Design review of the part built by this model. Coordinates are the model's own, in mm. Face numbers are marked on the shaded views. A direction names the side the tool comes from. Coordinates: 2 decimals unless noted, no trailing zeros. Order: outer loops, then holes, each group sorted by start corner. A loop starts at its lowest first (then second) coordinate and runs counter-clockwise, first axis right, second up. Notation, with made-up numbers: M 31,6.25 L 68,6.25 A14 ccw 68,22.25 Z; hole C -34,5.5 d7. An arc over 180 degrees is marked long. Use CSV: the item, a comma, the result in double quotes.
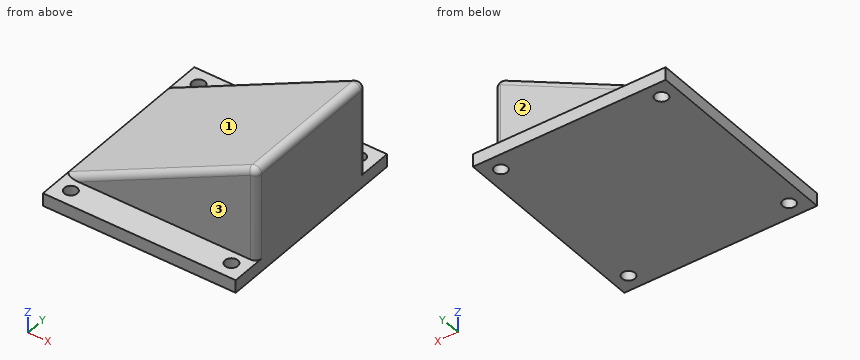
```python
from build123d import *

# Parameters (mm, degrees)
F0_W     = 30
F0_H     = 32
F1_DEPTH = 2
F2_R     = 1
F3_DEPTH = 2
F4_W     = 30
F4_H     = 23
F5_DEPTH = 15
F7_DEPTH = 23
F8_R     = 1


with BuildPart() as f1:
    # F0 (on Top) → F1 (new body)
    with BuildSketch(Plane.XY):
        Rectangle(F0_W, F0_H)
    extrude(amount=F1_DEPTH)

    # F2 (on face) → F3 (cut)
    with BuildSketch(Plane.XY.offset(2)):
        with Locations((12.5, 13.5)):
            Circle(F2_R)
        with Locations((-12.5, 13.5)):
            Circle(F2_R)
        with Locations((-12.5, -13.5)):
            Circle(F2_R)
        with Locations((12.5, -13.5)):
            Circle(F2_R)
    extrude(amount=-F3_DEPTH, mode=Mode.SUBTRACT)

    # F4 (on face) → F5 (join)
    with BuildSketch(Plane.XY.offset(2)):
        Rectangle(F4_W, F4_H)
    extrude(amount=F5_DEPTH)

    # F6 (on face) → F7 (cut)
    with BuildSketch(Plane.XZ.offset(11.5)):
        Polygon((-15, 2), (15, 17), (-15, 17), align=None)
    extrude(amount=-F7_DEPTH, mode=Mode.SUBTRACT)

    # F8
    f8_edges = [f1.edges().sort_by_distance(p)[0] for p in [
        (15, -11.5, 9.5),
        (15, 0, 17),
        (0, -11.5, 9.5),
        (15, 11.5, 9.5),
        (0, 11.5, 9.5),
    ]]
    fillet(f8_edges, radius=F8_R)


solid = f1.part
```
(1) Add section C-C on x = 12. Give the number of separate pieces and of enclosed holes in the cut face, and give its area (3 significant figures).
The answers:
separate pieces,"3"
enclosed holes,"0"
area,"367 mm2"
(2) For the marked faces 1, 2 and 3, list the 3-axis set-ups (+Z, -Z, +X, -X, +Y, -Y) from which the entire face can be reached by the end or side of a thin tool; tool diameter is ignored.
The answers:
face 1,"+Z, -X, +Y, -Y"
face 2,"+Z, +X, -X, +Y"
face 3,"+Z, +X, -X, -Y"
(3) Wall thickness on probe 1 along Y at (x, z) = (-12.5, 0.9); probe 2 along Y at (x, z) = (12.5, 8.5); probe 3 along Z at (x, y) = (6.5, -14): over which ranges is each line inside the solid? List them lowest first.
The answers:
probe 1,"y = -16 to -14.5, -12.5 to 12.5, 14.5 to 16"
probe 2,"y = -11.5 to 11.5"
probe 3,"z = 0 to 2"
(4) Add section B-B on y = -1.5. State the section outline as (x, z) points, and give its area (3 significant figures).
The answers:
outline,"M -15,0 L 15,0 L 15,15.38 A1 ccw 13.55,16.28 L -15,2 Z"
area,"284 mm2"
(5) Clearance check with flat-ended pins moving along their axes: P1, Ø6, axis at y = 2, z = 6.5, coming from the -X side; P2, Ø3, axis at x = -5.5, z = 7, coming from the +Y side; P3, Ø1.5, axis at x = 5.5, y = 6.5, coming from the +Z side (3 decimals). State where each tip first meets the part, or that it passes through.
The answers:
P1,"stops at x = -12"
P2,"stops at y = 11.5"
P3,"stops at z = 12.625"
(6) Add section A-A on y = 13.5. State the section outline as (x, z) points, and give its area (3 significant figures).
The answers:
outline,"M -15,0 L -13.5,0 L -13.5,2 L -15,2 Z; M -11.5,0 L 11.5,0 L 11.5,2 L -11.5,2 Z; M 13.5,0 L 15,0 L 15,2 L 13.5,2 Z"
area,"52.0 mm2"
(7) Add section D-D on y = -13. State the section outline as (x, z) points.
The answers:
outline,"M -15,0 L -13.37,0 L -13.37,2 L -15,2 Z; M -11.63,0 L 11.63,0 L 11.63,2 L -11.63,2 Z; M 13.37,0 L 15,0 L 15,2 L 13.37,2 Z"
